Design review of the part built by this model. Coordinates are the model's own, in mm. A direction names the side the tool comes from. Round coordinates to 2 decimals unless told otherwise and drop trailing zeros. Order: outer loops, then holes, each group sorted by start corner. A loop starts at its lowest first (then second) coordinate and runs counter-clockwise, first axis right, second up. Notation, with made-up numbers: M 36.25,16 L 84.25,16 A26 cw 84.25,38 Z; hole C 82,68.25 d4. An arc over 180 degrees is marked long. Use a Markdown table: item, result. Add a question column.
(1) For pin 1 (5 mm diameter, centred on x = 167, y = 90.5, fed in from -Z); pin 2 (10.5 mm diameter, centred on x = 48.5, y = 41, fed in from +Z), all flat-tipped, find the tip position at first contact; note any pin that passes through.
(2) The part is to be moulded in two halves that separate along Y. For faces 3 (the face through (789, 0, 13)), 4 (the face through (789, 150, 13)), 5 (the face through (68, 35, 23)), 6 (the face through (100, 74, 13)), say which applies: released by +Y, released by -Y, zero draft, split by the parting line, or undercut.
(3) Take a section at B-B (y = 83.5). Write out the cut boundary in (x, z), then the cut area to 3 significant figures.
(4) Take a section at A-A (z = 7.75). Write out the cut boundary in (x, y).
(5) Machinability: for faces 1 (the face through (72, 115, 23)), 2 (the face through (789, 76, 25.4)), which of the approach directions +Z, -Z, +X, -X, +Y, -Y give a long, thin tool a straight path to every point of the face, cutting with its end or side? Answer none if there is none.
(6) To check wall thickness, follow probe 1 along X at (y, z) = (100.5, 17); probe 2 along X at (y, z) = (89, 15.5). State the ranges of each line that lie inside material, in increasing order. Write a range as from..to.
```python
from build123d import *

# Parameters (mm, degrees)
SKETCH1_W           = 1600
SKETCH1_H           = 150
BOSS_EXTRUDE1_DEPTH = 25.4
CUT_EXTRUDE1_DEPTH  = 1608.216587769
SKETCH3_W           = 100
SKETCH3_H           = 80
CUT_EXTRUDE2_DEPTH  = 3
FILLET1_R           = 4


with BuildPart() as part:
    # Sketch1 → Boss-Extrude1 (new body)
    with BuildSketch(Plane.XY):
        with Locations((800, 75)):
            Rectangle(SKETCH1_W, SKETCH1_H)
    extrude(amount=BOSS_EXTRUDE1_DEPTH)

    # Sketch2 → Cut-Extrude1 (cut, through all)
    with BuildSketch(Plane.XY.offset(25.4)):
        Polygon((0, 52), (89, 52), (89, 35), (100, 35), (100, 115), (89, 115), (89, 98), (0, 98), align=None)
    extrude(amount=-CUT_EXTRUDE1_DEPTH, mode=Mode.SUBTRACT)

    # Sketch3 → Cut-Extrude2 (cut)
    with BuildSketch(Plane.XY.offset(25.4)):
        with Locations((50, 75)):
            Rectangle(SKETCH3_W, SKETCH3_H)
    extrude(amount=-CUT_EXTRUDE2_DEPTH, mode=Mode.SUBTRACT)

    # Fillet1
    fillet1_edges = [part.edges().sort_by_distance(p)[0] for p in [
        (44.5, 52, 22.4),
        (44.5, 98, 22.4),
    ]]
    fillet(fillet1_edges, radius=FILLET1_R)


solid = part.part
```
Verdict:
| question | item | result |
|---|---|---|
| 1 | pin 1 | stops at z = 0 |
| 1 | pin 2 | stops at z = 22.4 |
| 2 | face 3 | released by -Y |
| 2 | face 4 | released by +Y |
| 2 | face 5 | undercut |
| 2 | face 6 | undercut |
| 3 | outline | M 100,0 L 1600,0 L 1600,25.4 L 100,25.4 Z |
| 3 | area | 38,100 mm^2 |
| 4 | outline | M 0,0 L 1600,0 L 1600,150 L 0,150 L 0,98 L 89,98 L 89,115 L 100,115 L 100,35 L 89,35 L 89,52 L 0,52 Z |
| 5 | face 1 | +Z |
| 5 | face 2 | +Z, +X, -X, +Y, -Y |
| 6 | probe 1 | x = 0..89, 100..1600 |
| 6 | probe 2 | x = 100..1600 |
